from build123d import *

# Parameters (mm, degrees)
F0_R     = 5
F1_DEPTH = 1
F3_DEPTH = 2
F5_DEPTH = 2


with BuildPart() as f1:
    # F0 (on Top) → F1 (new body)
    with BuildSketch(Plane.XY):
        Circle(F0_R)
    extrude(amount=F1_DEPTH)

    # F2 (on Front) → F3 (join)
    with BuildSketch(Plane.XZ):
        Polygon((-2.4001505226, 4.9579590559), (-3.1682769768, 0.7939044153), (-2.0160870627, 0.7332628593), (0, 4.6908766963), (0, 11.689173989), (-1.0660358239, 11.689173989), (-2.1373701748, 11.1433994025), (-2.1373701748, 7.848540321), (-1.8341623945, 7.5049051084), (-2.7235720772, 5.4835192859), align=None)
        Polygon((0, 11.689173989), (0, 4.6908766963), (2.0160870627, 0.7332628593), (3.1682769768, 0.7939044153), (2.4001505226, 4.9579590559), (2.7235720772, 5.4835192859), (1.8341623945, 7.5049051084), (2.1373701748, 7.848540321), (2.1373701748, 11.1433994025), (1.0660358239, 11.689173989), align=None)
    extrude(amount=F3_DEPTH)

    # F4 (on face) → F5 (join)
    with BuildSketch(Plane.XY.offset(11.689173989)):
        with BuildLine():
            Line((0.7512930037, 0), (0, 0))
            Line((0, 0), (0, -2))
            Line((0, -2), (0.7512930037, -2))
            ThreePointArc((0.7512930037, -2), (0.9249655721, -1.8419500388), (1.0660358239, -1.6542238146))
            Line((1.0660358239, -1.6542238146), (1.0660358239, -0.3457761854))
            ThreePointArc((1.0660358239, -0.3457761854), (0.9249655721, -0.1580499612), (0.7512930037, 0))
        make_face()
        with BuildLine():
            Line((-0.7512930037, 0), (0, 0))
            Line((0, 0), (0.7512930037, 0))
            ThreePointArc((0.7512930037, 0), (0, 0.25077623), (-0.7512930037, 0))
        make_face()
        with BuildLine():
            Line((0, -2), (0, 0))
            Line((0, 0), (-0.7512930037, 0))
            ThreePointArc((-0.7512930037, 0), (-0.9249655721, -0.1580499612), (-1.0660358239, -0.3457761854))
            Line((-1.0660358239, -0.3457761854), (-1.0660358239, -1.6542238146))
            ThreePointArc((-1.0660358239, -1.6542238146), (-0.9249655721, -1.8419500388), (-0.7512930037, -2))
            Line((-0.7512930037, -2), (0, -2))
        make_face()
        with BuildLine():
            Line((0.7512930037, -2), (0, -2))
            Line((0, -2), (-0.7512930037, -2))
            ThreePointArc((-0.7512930037, -2), (0, -2.25077623), (0.7512930037, -2))
        make_face()
        with BuildLine():
            ThreePointArc((1.25077623, -1), (1.2037054138, -0.6600964044), (1.0660358239, -0.3457761854))
            Line((1.0660358239, -0.3457761854), (1.0660358239, -1.6542238146))
            ThreePointArc((1.0660358239, -1.6542238146), (1.2037054138, -1.3399035956), (1.25077623, -1))
        make_face()
        with BuildLine():
            Line((-1.0660358239, -1.6542238146), (-1.0660358239, -0.3457761854))
            ThreePointArc((-1.0660358239, -0.3457761854), (-1.25077623, -1), (-1.0660358239, -1.6542238146))
        make_face()
    extrude(amount=F5_DEPTH)


solid = f1.part
Input: part model. Units: mm. Frame: model coordinates. A direction names the side the tool comes from. Coordinates: 2 decimals unless noted, no trailing zeros. Loops run counter-clockwise (first coordinate to the right, second up) from the corner with the lowest first, then second, coordinate; pieces in that order, holes last. Notation, with made-up numbers: (-21.5, -37) -> (-6.5, -37) arc R12 ccw to (-6.5, -25) -> close; hole circle Ø8 at (86, 75). An arc over 180 degrees is marked (long way). One line per item, written item: value.
(1) Pin query (flat end, axial travel): pin 1 Ø4 at (y, z) = (1.5, 4.5) entering from -X; pin 2 Ø3 at (x, z) = (-1, 7) entering from -Y; pin 3 Ø2 at (y, z) = (-1, 10) entering from +X. Return the tip coordinate at first contact, or that it passes through.
Answer below:
pin 1: stops at x = -2.73
pin 2: stops at y = -2
pin 3: stops at x = 2.14
(2) Cut plane B-B (z = 10.25). Output: boundary loops of the cut face in (x, y), then the cut area to 3 significant figures.
Answer below:
outline: (-2.14, -2) -> (2.14, -2) -> (2.14, 0) -> (-2.14, 0) -> close
area: 8.55 mm2
(3) Ray query, line 1 along Z through (x, y) = (-1, -0.5); line 2 along Y through (x, z) = (0.5, 4); line 3 along Z through (x, y) = (-0.25, 0.75). Return the intervals inside material, ascending.
Answer below:
line 1: z = 0 to 1, 2.73 to 13.69
line 2: y = -2 to 0
line 3: z = 0 to 1
(4) Set-up query: faces 4 (the face through (0, 0, 6)), 5 (the face through (-0.953, -0.986, 2.82)), 6 (the face through (2.137, -1, 9)). Return all of +Z, -Z, +X, -X, +Y, -Y with unobstructed straight access to the full face (end or side cutting, diameter ignored); none if empty.
Answer below:
face 4: +X, -X, +Y
face 5: +Y, -Y
face 6: +Z, +X, +Y, -Y
(5) Cut plane C-C (x = -4). Output: boundary loops of the cut face in (y, z).
Answer below:
outline: (-3, 0) -> (3, 0) -> (3, 1) -> (-3, 1) -> close
(6) Cut plane A-A (x = -0.5). Output: boundary loops of the cut face in (y, z), then the cut area to 3 significant figures.
Answer below:
outline: (-4.97, 0) -> (4.97, 0) -> (4.97, 1) -> (-4.97, 1) -> close; (-2.15, 11.69) -> (-2, 11.69) -> (-2, 3.71) -> (0, 3.71) -> (0, 11.69) -> (0.15, 11.69) -> (0.15, 13.69) -> (-2.15, 13.69) -> close
area: 30.5 mm2
(7) Draft query along Z for faces 1 (the face through (-2.27, -0.99, 6.51)), 2 (the face through (-2.137, -1, 10)), 3 (the face through (0, 0, 0)). Return one class per face: pulls with the +Z half, pulls with the -Z half, needs draft (parallel to the pull), parting line crosses it, or undercut.
Answer below:
face 1: undercut
face 2: needs draft
face 3: pulls with the -Z half
(8) Cut plane D-D (x = 1.5). Output: boundary loops of the cut face in (y, z).
Answer below:
outline: (-4.77, 0) -> (4.77, 0) -> (4.77, 1) -> (-4.77, 1) -> close; (-2, 1.75) -> (0, 1.75) -> (0, 11.47) -> (-2, 11.47) -> close
